Design review of the part shown in the three views and the two pictorial views. Dimensions are in mm from the part's minimum x, y and z. A direction names the side the tool comes from. Round coordinates to 2 decimals unless told otherwise and drop trailing zeros. Loops run counter-clockwise (first coordinate to the right, second up) from the corner with the lowest first, then second, coordinate; pieces in that order, holes last.
1. Consider section A-A on y = 26. State the section outline as (x, z) points (1 decimal).
2. To check wall thickness, follow line 1 along Y through (x, z) = (107, 2); line 2 along X through (y, z) = (13.5, 8); line 3 along Y through (x, z) = (5.5, 41). State the ranges of each line that lie inside material, in increasing order.
3. Clearance check with flat-ended pins moving along their axes: pin 1 Ø22 at (x, z) = (110.5, 10.5) entering from -Y; pin 2 Ø23 at (x, y) = (64.46, 28.42) entering from +Z; pin 3 Ø12.5 at (y, z) = (13, 18) entering from +X; pin 4 Ø5 at (x, z) = (8, 44) entering from -Y. State where each tip first meets the part, or that it passes through.
4. Tool access review of the marked faces 4, 5, 6, 7 and 8: name each direction out of +Z, -Z, +X, -X, +Y, -Y from which nothing blocks a thin tool from reaching the whole face with its end or side.
5. Consider section D-D on x = 15.5. State the section outline as (y, z) points (1 decimal).
6. Draft analysis for pull direction X (two halves, no side actions). For the marked faces 1, 2 and 3, state which applies: released by +X, released by -X, zero draft, split by the parting line, or undercut.
7. Consider section C-C on z = 17.5. State the section outline as (x, y) points (1 decimal), then the cut area to 3 significant figures.
8. Consider section B-B on x = 59. State the section outline as (y, z) points (1 decimal), then the cut area to 3 significant figures.
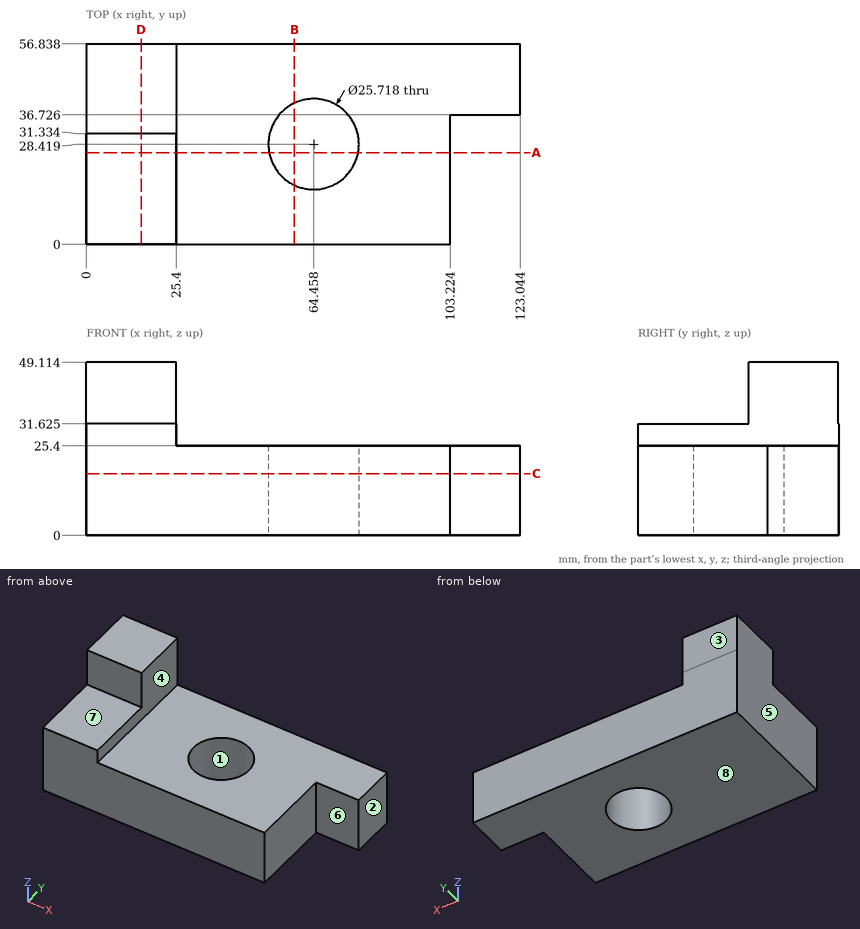
Resolved:
1. outline: (0, 0) - (51.8, 0) - (51.8, 25.4) - (25.4, 25.4) - (25.4, 31.6) - (0, 31.6) - close; (77.1, 0) - (103.2, 0) - (103.2, 25.4) - (77.1, 25.4) - close
2. line 1: y = 36.73 to 56.84
2. line 2: x = 0 to 103.22
2. line 3: y = 31.33 to 56.84
3. pin 1: stops at y = 0
3. pin 2: passes through
3. pin 3: stops at x = 103.22
3. pin 4: stops at y = 31.33
4. face 4: +Z, +X, +Y, -Y
4. face 5: +Z, -Z, -X, +Y, -Y
4. face 6: +Z, -Z, +X, -Y
4. face 7: +Z, +X, -X, -Y
4. face 8: -Z, +X, -X, +Y, -Y
5. outline: (0, 0) - (56.8, 0) - (56.8, 49.1) - (31.3, 49.1) - (31.3, 31.6) - (0, 31.6) - close
6. face 1: undercut
6. face 2: released by +X
6. face 3: zero draft
7. outline: (0, 0) - (103.2, 0) - (103.2, 36.7) - (123, 36.7) - (123, 56.8) - (0, 56.8) - close; hole circle Ø25.7 at (64.5, 28.4)
7. area: 5,750 mm2
8. outline: (0, 0) - (16.8, 0) - (16.8, 25.4) - (0, 25.4) - close; (40.1, 0) - (56.8, 0) - (56.8, 25.4) - (40.1, 25.4) - close
8. area: 852 mm2
